For this review, use the dimensioned drawing (mm, ordinates from the lowest corner) and the shaded views. Coordinates: 2 decimals unless noted, no trailing zeros. Loops run counter-clockwise (first coordinate to the right, second up) from the corner with the lowest first, then second, coordinate; pieces in that order, holes last. Notation, with made-up numbers: (83.25, 56.5) - (97.25, 56.5) arc R25 cw to (97.25, 68.5) - close; hole circle Ø3 at (12, -17.75). An arc over 180 degrees is marked (long way). Use one line per item in the form item = value. Start each with the question number.
(1) Add section D-D (y = 4.6). State the section outline as (x, z) points, plus the area to 3 significant figures.
(2) For L1, parallel to Y at x = 3, z = 0.55; L2, parallel to Y at x = 2.25, z = 0.5; L3, parallel to X at y = 4.6, z = 1.1, list the stretches that pass through material, from the lowest coordinate up.
(3) The part is to be moulded in two halves that separate along Y. For the marked faces 1, 2 and 3, say which applies: pulls with the +Y half, pulls with the -Y half, needs draft (parallel to the pull), parting line crosses it, or undercut.
(4) Add section C-C (y = 0.75). State the section outline as (x, z) points.
(5) Add section B-B (x = 4). State the section outline as (y, z) points, plus the area to 3 significant figures.
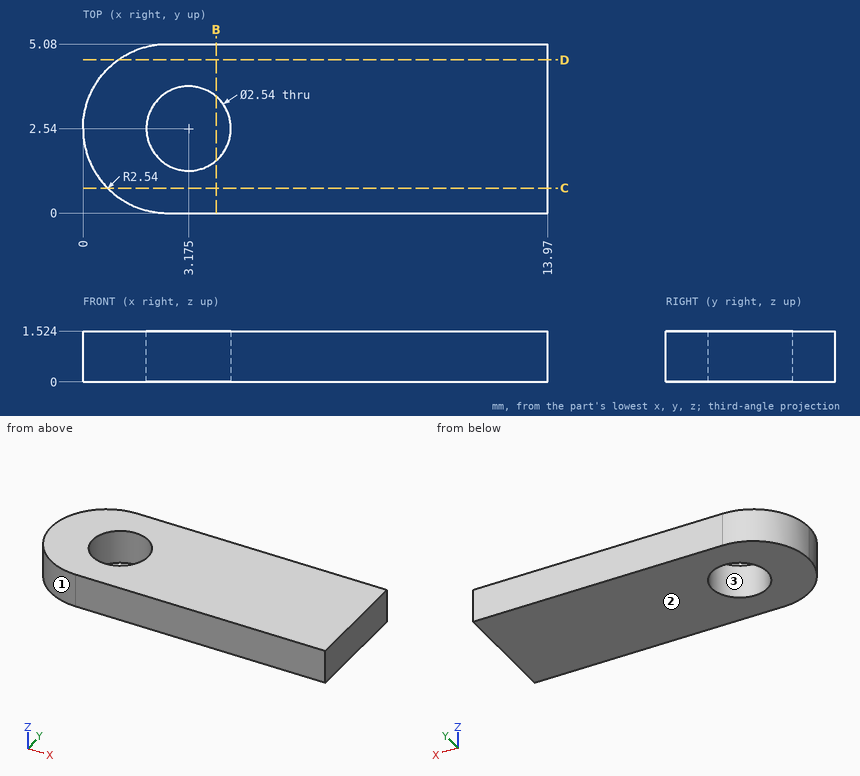
Computed values:
q1.outline = (1.05, 0) - (13.97, 0) - (13.97, 1.52) - (1.05, 1.52) - close
q1.area = 19.7 mm^2
q2.L1 = 0 to 1.28, 3.8 to 5.08
q2.L2 = 0.02 to 1.67, 3.41 to 5.06
q2.L3 = 1.05 to 13.97
q3.face_1 = pulls with the -Y half
q3.face_2 = needs draft
q3.face_3 = undercut
q4.outline = (0.74, 0) - (13.97, 0) - (13.97, 1.52) - (0.74, 1.52) - close
q5.outline = (0, 0) - (1.57, 0) - (1.57, 1.52) - (0, 1.52) - close; (3.51, 0) - (5.08, 0) - (5.08, 1.52) - (3.51, 1.52) - close
q5.area = 4.80 mm^2
